Autodesk Inventor part; units mm, degrees
ref_plane "Work Plane1" through (0, 0, 1.825) normal (0, 0, 1) x (1, 0, 0)
ref_plane "YZ Plane" through (0, 0, 0) normal (1, 0, 0) x (0, 1, 0)
ref_plane "XZ Plane" through (0, 0, 0) normal (0, 1, 0) x (-1, 0, 0)
ref_plane "Work Plane1" through (0, 0, 1.825) normal (0, 0, 1) x (1, 0, 0)
sketch "Sketch1" plane through (0, 0, 1.825) normal (0, 0, 1) x (1, 0, 0)
  line L0 (5.7, 2) -> (-19.7, 2)
  line L1 (5.7, 4.5) -> (5.7, 2)
  line L2 (-0.5, 13.7) -> (-5.2, 13.7)
  line L3 (-8.8, 6.3) -> (-8.8, 13.7)
  line L4 (-13.5, 4.5) -> (-19.7, 4.5)
  line L5 (5.7, 4.5) -> (-0.5, 4.5)
  line L6 (-5.2, 6.3) -> (-5.2, 13.7)
  line L7 (-8.8, 13.7) -> (-13.5, 13.7)
  line L8 (-19.7, 4.5) -> (-19.7, 2)
  line L9 (-0.5, 4.5) -> (-0.5, 13.7)
  arc A0 (-8.8, 6.3) -> (-5.2, 6.3) centre (-7, 6.3) ccw
  line L10 (-13.5, 4.5) -> (-13.5, 13.7)
extrude "Extrusion3" add sketch "Sketch1" along normal blind 6.35
sketch "Sketch2" plane through (-19.7, 2, 1.825) normal (0, -1, 0) x (1, 0, 0)
  line L0 (0.2, 0) -> (0.2, 6.175)
  line L1 (0.2, 6.175) -> (25.4, 6.175)
  line L2 (25.4, 6.175) -> (39.2, 6.175)
  line L3 (39.2, 6.175) -> (39.2, -9.825)
  line L4 (39.2, -9.825) -> (0.2, -9.825)
  line L5 (0.2, -9.825) -> (0.2, 0)
extrude "Extrusion2" add sketch "Sketch2" along normal blind 2
hole "Hole2" at (-16.5, 0, 5) direction (0, 1, 0) diameter 3 depth 4.5
sketch "Sketch3" plane through (0, 0, 0) normal (0, 1, 0) x (-1, 0, 0)
  point P0 (16.5, 5)
hole "Hole1" at (2.5, 0, 5) direction (0, 1, 0) diameter 3 depth 4.5
sketch "Sketch5" plane through (-19.7, 2, 1.825) normal (0, 1, 0) x (1, 0, 0)
  line L0 (31, -5.975) -> (39, -5.975)
  line L1 (39, -5.975) -> (39, 9.625)
  line L2 (31, 9.625) -> (31, -5.975)
  line L3 (39, 9.625) -> (31, 9.625)
extrude "Extrusion1" add sketch "Sketch5" along normal blind 10
sketch "Sketch4" plane through (0, 0, 0) normal (0, 1, 0) x (-1, 0, 0)
  point P0 (-2.5, 5)
properties part number "Endstop"
Model file for the job. Use its own axes, mm. A direction names the side the tool comes from. Give positions to 0.01 mm unless a question says otherwise; leave off trailing zeros. Order: outer loops, then holes, each group sorted by start corner. A loop starts at its lowest first (then second) coordinate and runs counter-clockwise, first axis right, second up. Notation, with made-up numbers: M 30.5,46 L 88.5,46 A12 ccw 88.5,56 Z; hole C -14.5,83 d1. An arc over 180 degrees is marked long. Put each result on its own line as item: value. Start each with the question number.
(1) Tool access for faces 5 (the face through (-13.5, 9, 5)), 6 (the face through (19.3, 7, 0)), 7 (the face through (5.7, 3, 5)), 8 (the face through (15, 7, 7.8)), 9 (the face through (-19.5, 1, 0)): list every direction of +Z, -Z, +X, -X, +Y, -Y with a clear straight run to the whole face (end or side of a thin tool).
(2) Band-saw the part on D-D on y = 8.5. Give the cut face in (x, z) (3 decimals), then the cut area to 3 significant figures.
(3) Band-saw the part on C-C on z = 5.75. Give the cut face in (x, y), then the cut area to 3 significant figures.
(4) Drill centre lines: L1, parallel to X at y = 1.1, z = 5; L2, parallel to X at y = 8.25, z = 5; L3, parallel to Z at x = -16.5, y = 0.9. Where is each one in solid material? Low to high. Write a range as [from, to].
(5) Pull direction Z, two halves, no side cores. Call faces 1 (the face through (-3, 13.7, 5)), 2 (the face through (-17.51, 2.28, 6.11)), 3 (the face through (0, 1, 8)), 4 (the face through (-4, 7, 1.825)): released by +Z, released by -Z, zero draft, split by the parting line, or undercut.
(6) Band-saw the part on B-B on y = 13.25. Give the cut face in (x, z) (3 decimals).
(7) Pin check, flat tips, straight feed: pin 1 Ø2 at (x, z) = (-13, -4.5) entering from -Y; pin 2 Ø3 at (x, z) = (2, 5) entering from +Y; pin 3 Ø6.5 at (x, z) = (15.5, 1.5) entering from +Y; pin 4 Ø3 at (y, z) = (9.5, 5) entering from -X. Stop position of each tip, or through.
(8) Band-saw the part on A-A on x = -16.5. Give the cut face in (y, z) (3 decimals).
Results below:
1. face 5: +Z, -Z, -X, +Y
1. face 6: +Z, -Z, +X, +Y
1. face 7: +Z, -Z, +Y
1. face 8: +Z, +X, +Y
1. face 9: +Z, -Z, -X, -Y
2. outline: M -13.5,1.825 L -8.8,1.825 L -8.8,8.175 L -13.5,8.175 Z; M -5.2,1.825 L -0.5,1.825 L -0.5,8.175 L -5.2,8.175 Z; M 11.3,-7.8 L 19.3,-7.8 L 19.3,7.8 L 11.3,7.8 Z
2. area: 184 mm2
3. outline: M -19.7,2 L -19.5,2 L -19.5,0 L -17.8,0 L -17.8,4.5 L -19.7,4.5 Z; M -15.2,0 L 1.2,0 L 1.2,4.5 L -0.5,4.5 L -0.5,13.7 L -5.2,13.7 L -5.2,6.3 A1.8 cw -8.8,6.3 L -8.8,13.7 L -13.5,13.7 L -13.5,4.5 L -15.2,4.5 Z; M 3.8,0 L 19.5,0 L 19.5,2 L 19.3,2 L 19.3,12 L 11.3,12 L 11.3,2 L 5.7,2 L 5.7,4.5 L 3.8,4.5 Z
3. area: 286 mm2
4. L1: x = [-19.5, -18], [-15, 1], [4, 19.5]
4. L2: x = [-13.5, -8.8], [-5.2, -0.5], [11.3, 19.3]
4. L3: z = [-8, 3.5], [6.5, 8]
5. face 1: zero draft
5. face 2: undercut
5. face 3: released by +Z
5. face 4: released by -Z
6. outline: M -13.5,1.825 L -8.8,1.825 L -8.8,8.175 L -13.5,8.175 Z; M -5.2,1.825 L -0.5,1.825 L -0.5,8.175 L -5.2,8.175 Z
7. pin 1: stops at y = 0
7. pin 2: stops at y = 4.5
7. pin 3: stops at y = 12
7. pin 4: stops at x = -13.5
8. outline: M 0,-8 L 2,-8 L 2,1.825 L 4.5,1.825 L 4.5,3.5 L 0,3.5 Z; M 0,6.5 L 4.5,6.5 L 4.5,8.175 L 2,8.175 L 2,8 L 0,8 Z
